```python
from build123d import *

# Parameters (mm, degrees)
SKETCH1_W               = 120
SKETCH1_H               = 25
COUPON_120X25_DEPTH     = 4
DIAMETER_1P8_START      = -0.1
SKETCH2_R               = 0.9
DIAMETER_1P8_DEPTH      = 4.2
DIAMETER_1P9_START      = -0.1
SKETCH3_R               = 0.95
DIAMETER_1P9_DEPTH      = 4.2
DIAMETER_2_START        = -0.1
SKETCH4_R               = 1
DIAMETER_2_DEPTH        = 4.2
DIAMETER_2P1_START      = -0.1
SKETCH5_R               = 1.05
DIAMETER_2P1_DEPTH      = 4.2
DIAMETER_2P2_START      = -0.1
SKETCH6_R               = 1.1
DIAMETER_2P2_DEPTH      = 4.2
DIAMETER_2P3_START      = -0.1
SKETCH7_R               = 1.15
DIAMETER_2P3_DEPTH      = 4.2
DIAMETER_3P2_START      = -0.1
SKETCH8_R               = 1.6
DIAMETER_3P2_DEPTH      = 4.2
DIAMETER_3P4_START      = -0.1
SKETCH9_R               = 1.7
DIAMETER_3P4_DEPTH      = 4.2
DIAMETER_8P2_START      = -0.1
SKETCH10_R              = 4.1
DIAMETER_8P2_DEPTH      = 4.2
DIAMETER_8P4_START      = -0.1
SKETCH11_R              = 4.2
DIAMETER_8P4_DEPTH      = 4.2
DIAMETER_8P6_START      = -0.1
SKETCH12_R              = 4.3
DIAMETER_8P6_DEPTH      = 4.2
ORIENTATION_NOTCH_START = -0.1
SKETCH13_W              = 4
SKETCH13_H              = 4
ORIENTATION_NOTCH_DEPTH = 4.2


with BuildPart() as part:
    # Sketch1 → Coupon_120x25 (new body)
    with BuildSketch(Plane.XY):
        Rectangle(SKETCH1_W, SKETCH1_H)
    extrude(amount=COUPON_120X25_DEPTH)

    # Sketch2 → Diameter_1p8 (cut)
    with BuildSketch(Plane.XY.offset(DIAMETER_1P8_START)):
        with Locations(Location((-50, 0, 0), (0, 0, 180))):
            Circle(SKETCH2_R)
    extrude(amount=DIAMETER_1P8_DEPTH, mode=Mode.SUBTRACT)

    # Sketch3 → Diameter_1p9 (cut)
    with BuildSketch(Plane.XY.offset(DIAMETER_1P9_START)):
        with Locations(Location((-40, 0, 0), (0, 0, 180))):
            Circle(SKETCH3_R)
    extrude(amount=DIAMETER_1P9_DEPTH, mode=Mode.SUBTRACT)

    # Sketch4 → Diameter_2 (cut)
    with BuildSketch(Plane.XY.offset(DIAMETER_2_START)):
        with Locations(Location((-30, 0, 0), (0, 0, 180))):
            Circle(SKETCH4_R)
    extrude(amount=DIAMETER_2_DEPTH, mode=Mode.SUBTRACT)

    # Sketch5 → Diameter_2p1 (cut)
    with BuildSketch(Plane.XY.offset(DIAMETER_2P1_START)):
        with Locations(Location((-20, 0, 0), (0, 0, 180))):
            Circle(SKETCH5_R)
    extrude(amount=DIAMETER_2P1_DEPTH, mode=Mode.SUBTRACT)

    # Sketch6 → Diameter_2p2 (cut)
    with BuildSketch(Plane.XY.offset(DIAMETER_2P2_START)):
        with Locations(Location((-10, 0, 0), (0, 0, 180))):
            Circle(SKETCH6_R)
    extrude(amount=DIAMETER_2P2_DEPTH, mode=Mode.SUBTRACT)

    # Sketch7 → Diameter_2p3 (cut)
    with BuildSketch(Plane.XY.offset(DIAMETER_2P3_START)):
        with Locations(Location((0, 0, 0), (0, 0, 180))):
            Circle(SKETCH7_R)
    extrude(amount=DIAMETER_2P3_DEPTH, mode=Mode.SUBTRACT)

    # Sketch8 → Diameter_3p2 (cut)
    with BuildSketch(Plane.XY.offset(DIAMETER_3P2_START)):
        with Locations(Location((10, 0, 0), (0, 0, 180))):
            Circle(SKETCH8_R)
    extrude(amount=DIAMETER_3P2_DEPTH, mode=Mode.SUBTRACT)

    # Sketch9 → Diameter_3p4 (cut)
    with BuildSketch(Plane.XY.offset(DIAMETER_3P4_START)):
        with Locations(Location((20, 0, 0), (0, 0, 180))):
            Circle(SKETCH9_R)
    extrude(amount=DIAMETER_3P4_DEPTH, mode=Mode.SUBTRACT)

    # Sketch10 → Diameter_8p2 (cut)
    with BuildSketch(Plane.XY.offset(DIAMETER_8P2_START)):
        with Locations(Location((30, 0, 0), (0, 0, 180))):
            Circle(SKETCH10_R)
    extrude(amount=DIAMETER_8P2_DEPTH, mode=Mode.SUBTRACT)

    # Sketch11 → Diameter_8p4 (cut)
    with BuildSketch(Plane.XY.offset(DIAMETER_8P4_START)):
        with Locations(Location((40, 0, 0), (0, 0, 180))):
            Circle(SKETCH11_R)
    extrude(amount=DIAMETER_8P4_DEPTH, mode=Mode.SUBTRACT)

    # Sketch12 → Diameter_8p6 (cut)
    with BuildSketch(Plane.XY.offset(DIAMETER_8P6_START)):
        with Locations(Location((50, 0, 0), (0, 0, 180))):
            Circle(SKETCH12_R)
    extrude(amount=DIAMETER_8P6_DEPTH, mode=Mode.SUBTRACT)

    # Sketch13 → Orientation_Notch (cut)
    with BuildSketch(Plane.XY.offset(ORIENTATION_NOTCH_START)):
        with Locations((-58, -10.5)):
            Rectangle(SKETCH13_W, SKETCH13_H)
    extrude(amount=ORIENTATION_NOTCH_DEPTH, mode=Mode.SUBTRACT)


solid = part.part
```
Geometry: final body of the model. Coordinates: model frame, mm. A direction names the side the tool comes from. Round coordinates to 2 decimals unless told otherwise and drop trailing zeros. Write each loop counter-clockwise with the first axis right and the second up, starting at its lowest first coordinate (ties: lowest second). Pieces come first, ordered by that corner, then holes.
Item 1: Section query C-C (x = 40). Return loops of the section in (y, z), plus the area to 3 significant figures.
Item 2: Mould query, pull axis Y, two halves, no side actions, for faces 1 (the face through (0.91, 0.7, 1.97)), 2 (the face through (-1, 12.5, 2)), 3 (the face through (-56, -11, 2)). Classes: +Y half, -Y half, draft (parallel to the pull), parting line (faces both ways), or undercut.
Item 3: Section query B-B (z = 2.9). Give the number of separate pieces and of enclosed holes in the cut face, plus the area to 3 significant figures.
Item 4: Section query A-A (x = 0). Return loops of the section in (y, z), plus the area to 3 significant figures.
Item 5: Pin query (flat end, axial travel): P1, Ø2, axis at x = -50, y = 0, coming from the +Z side; P2, Ø2, axis at x = -57.5, z = 2, coming from the -Y side. Return the tip coordinate at first contact, or that it passes through.
Item 6: Set-up query: faces 4 (the face through (-58, -8.5, 2)), 5 (the face through (11.6, -0.07, 1.97)). Return all of +Z, -Z, +X, -X, +Y, -Y with unobstructed straight access to the full face (end or side cutting, diameter ignored); none if empty.
Item 7: Material intervals for L1, parallel to X at y = -3.25, z = 0.5; L2, parallel to Y at x = -20, z = 2.1; L3, parallel to X at y = -1.75, z = 3.05, sorted ascending.
Completed:
1. outline: (-12.5, 0) - (-4.2, 0) - (-4.2, 4) - (-12.5, 4) - close; (4.2, 0) - (12.5, 0) - (12.5, 4) - (4.2, 4) - close
1. area: 66.4 mm2
2. face 1: undercut
2. face 2: +Y half
2. face 3: draft
3. separate pieces: 1
3. enclosed holes: 11
3. area: 2,780 mm2
4. outline: (-12.5, 0) - (-1.15, 0) - (-1.15, 4) - (-12.5, 4) - close; (1.15, 0) - (12.5, 0) - (12.5, 4) - (1.15, 4) - close
4. area: 90.8 mm2
5. P1: stops at z = 4
5. P2: stops at y = -8.5
6. face 4: +Z, -Z, -X, -Y
6. face 5: +Z, -Z
7. L1: x = -60 to 27.5, 32.5 to 37.34, 42.66 to 47.18, 52.82 to 60
7. L2: y = -12.5 to -1.05, 1.05 to 12.5
7. L3: x = -60 to 26.29, 33.71 to 36.18, 43.82 to 46.07, 53.93 to 60
